from build123d import *

# Parameters (mm, degrees)
SKETCH1_W           = 118
SKETCH1_H           = 82
BOSS_EXTRUDE1_DEPTH = 2
SKETCH3_R           = 1.5
CUT_EXTRUDE5_DEPTH  = 10
SKETCH4_R           = 1.6
CUT_EXTRUDE6_DEPTH  = 10
SKETCH7_R           = 1
SKETCH7_W           = 1.5
SKETCH7_H           = 3.5
CUT_EXTRUDE7_DEPTH  = 10
SKETCH5_W           = 22.5
SKETCH5_H           = 12
CUT_EXTRUDE8_DEPTH  = 10


with BuildPart() as part:
    # Sketch1 → Boss-Extrude1 (new body)
    with BuildSketch(Plane(origin=(0, 0, 0), x_dir=(1, 0, 0), z_dir=(0, 1, 0))):
        Rectangle(SKETCH1_W, SKETCH1_H)
    extrude(amount=BOSS_EXTRUDE1_DEPTH)

    # Sketch3 → Cut-Extrude5 (cut)
    with BuildSketch(Plane(origin=(0, 2, 0), x_dir=(1, 0, 0), z_dir=(0, 1, 0))):
        with Locations(Location((-57, 0, 0), (0, 0, 270))):
            Circle(SKETCH3_R)
        with Locations(Location((57, 0, 0), (0, 0, 90))):
            Circle(SKETCH3_R)
    extrude(amount=-CUT_EXTRUDE5_DEPTH, mode=Mode.SUBTRACT)

    # Sketch4 → Cut-Extrude6 (cut)
    with BuildSketch(Plane.XZ):
        with Locations(Location((-2.4, 37.960584027, 0), (0, 0, 270))):
            Circle(SKETCH4_R)
        with Locations(Location((-54.8, 32.860584027, 0), (0, 0, 270))):
            Circle(SKETCH4_R)
        with Locations(Location((-4, -10.339415973, 0), (0, 0, 270))):
            Circle(SKETCH4_R)
        with Locations(Location((-54.8, 4.960584027, 0), (0, 0, 270))):
            Circle(SKETCH4_R)
    extrude(amount=-CUT_EXTRUDE6_DEPTH, mode=Mode.SUBTRACT)

    # Sketch7 → Cut-Extrude7 (cut)
    with BuildSketch(Plane(origin=(0, 2, 0), x_dir=(1, 0, 0), z_dir=(0, 1, 0))):
        with Locations((24.125, -24.85)):
            Circle(SKETCH7_R)
        with Locations(Location((51.375, -24.85, 0), (0, 0, 270))):
            Circle(SKETCH7_R)
        with Locations((25.75, -24.85)):
            Rectangle(SKETCH7_W, SKETCH7_H)
    extrude(amount=-CUT_EXTRUDE7_DEPTH, mode=Mode.SUBTRACT)

    # Sketch5 → Cut-Extrude8 (cut)
    with BuildSketch(Plane(origin=(0, 2, 0), x_dir=(1, 0, 0), z_dir=(0, 1, 0))):
        with Locations((37.75, -24.85)):
            Rectangle(SKETCH5_W, SKETCH5_H)
    extrude(amount=-CUT_EXTRUDE8_DEPTH, mode=Mode.SUBTRACT)


solid = part.part
Here's how the part is built. I have some questions about the finished solid (model axes, mm). Coordinates: 2 decimals unless noted, no trailing zeros. Order: outer loops, then holes, each group sorted by start corner. A loop starts at its lowest first (then second) coordinate and runs counter-clockwise, first axis right, second up. Notation, with made-up numbers: (13, -12.75) -> (33, -12.75) arc R34 ccw to (33, 21.25) -> close; hole circle Ø9 at (89.5, 87.5). An arc over 180 degrees is marked (long way). Answer in a Markdown table with one row per item.
(1) Please list where these lines run through material, in increasing order: probe 1 along X at (y, z) = (0.8, 0); probe 2 along Z at (x, y) = (39.5, 0.85); probe 3 along X at (y, z) = (1.15, 23.5).
Answer key:
| item | result |
|---|---|
| probe 1 | -59 to -58.5, -55.5 to 55.5, 58.5 to 59 |
| probe 2 | -41 to 18.85, 30.85 to 41 |
| probe 3 | -59 to 25, 49 to 59 |
(2) Will these pins go through, and if not, where does the flat tip stop? pin 1 Ø3.5 at (x, z) = (-2.4, 37.96) entering from -Y; pin 2 Ø2.5 at (x, z) = (-4, -10.34) entering from -Y.
Answer key:
| item | result |
|---|---|
| pin 1 | y = 0 |
| pin 2 | through |
(3) I want a section at A-A on z = 0. List the corners of the cut face in (x, y) for me.
Answer key:
| item | result |
|---|---|
| outline | (-59, 0) -> (-58.5, 0) -> (-58.5, 2) -> (-59, 2) -> close; (-55.5, 0) -> (55.5, 0) -> (55.5, 2) -> (-55.5, 2) -> close; (58.5, 0) -> (59, 0) -> (59, 2) -> (58.5, 2) -> close |
(4) I want a section at C-C on z = 32.5. List the corners of the cut face in (x, y) for me, then the cut area to 3 significant figures.
Answer key:
| item | result |
|---|---|
| outline | (-59, 0) -> (-56.36, 0) -> (-56.36, 2) -> (-59, 2) -> close; (-53.24, 0) -> (59, 0) -> (59, 2) -> (-53.24, 2) -> close |
| area | 230 mm^2 |
(5) I want a section at B-B on x = 57. List the corners of the cut face in (y, z) for me, then the cut area to 3 significant figures.
Answer key:
| item | result |
|---|---|
| outline | (0, -41) -> (2, -41) -> (2, -1.5) -> (0, -1.5) -> close; (0, 1.5) -> (2, 1.5) -> (2, 41) -> (0, 41) -> close |
| area | 158 mm^2 |
(6) I want a section at D-D on y = 1.15. Count the separate pieces of the cut face and the enclosed holes in it, then the cut area to 3 significant figures.
Answer key:
| item | result |
|---|---|
| separate pieces | 1 |
| enclosed holes | 8 |
| area | 9,350 mm^2 |
(7) Thinking about a two-plate mould opening in X: for faces 1 (the face through (-55.513, 1.014, -0.195)), 2 (the face through (-1, 2, -1)), which applies, +X half, -X half, draft (parallel to the pull), parting line (faces both ways), or undercut?
Answer key:
| item | result |
|---|---|
| face 1 | undercut |
| face 2 | draft |
